For this review, use the dimensioned drawing (mm, ordinates from the lowest corner) and the shaded views. A direction names the side the tool comes from. Give positions to 0.01 mm unless a question says otherwise; leave off trailing zeros. Order: outer loops, then holes, each group sorted by start corner. A loop starts at its lowest first (then second) coordinate and runs counter-clockwise, first axis right, second up. Notation, with made-up numbers: M -20,-32.75 L -9,-32.75 A9 ccw -9,-15.75 Z; hole C -27.75,38 d3. An arc over 180 degrees is marked long. Use CSV: the item, a comma, the result in double quotes. Start each with the question number.
(1) Consider section A-A (z = 10.16). Write out the cut boundary in (x, y), and give its area (3 significant figures).
(2) Wall thickness on L1, parallel to Z at x = 2.5, y = 1; L2, parallel to X at y = 4.05, z = 6.35; L3, parallel to X at y = 1.15, z = 10.16: over which ranges is each line inside the solid? List them lowest first. Write a range as from..to.
(3) Draft analysis for pull direction X (two halves, no side actions). For the marked faces 1, 2 and 3, state which applies: pulls with the +X half, pulls with the -X half, needs draft (parallel to the pull), parting line crosses it, or undercut.
(4) Consider section B-B (x = 17.25). Write out the cut boundary in (y, z), and give its area (3 significant figures).
(5) Clearance check with flat-ended pins moving along their axes: P1, Ø1.6, axis at x = 10.5, z = 7, coming from the +Y side; P2, Ø8, axis at x = 4.5, z = 11, coming from the +Y side. State where each tip first meets the part, or that it passes through.
(6) Tool access review of the marked faces 4 and 5: name each direction out of +Z, -Z, +X, -X, +Y, -Y from which nothing blocks a thin tool from reaching the whole face with its end or side.
(7) Consider section D-D (x = 14.25). Write out the cut boundary in (y, z), and give its area (3 significant figures).
(8) Consider section C-C (y = 1.75). Write out the cut boundary in (x, z).
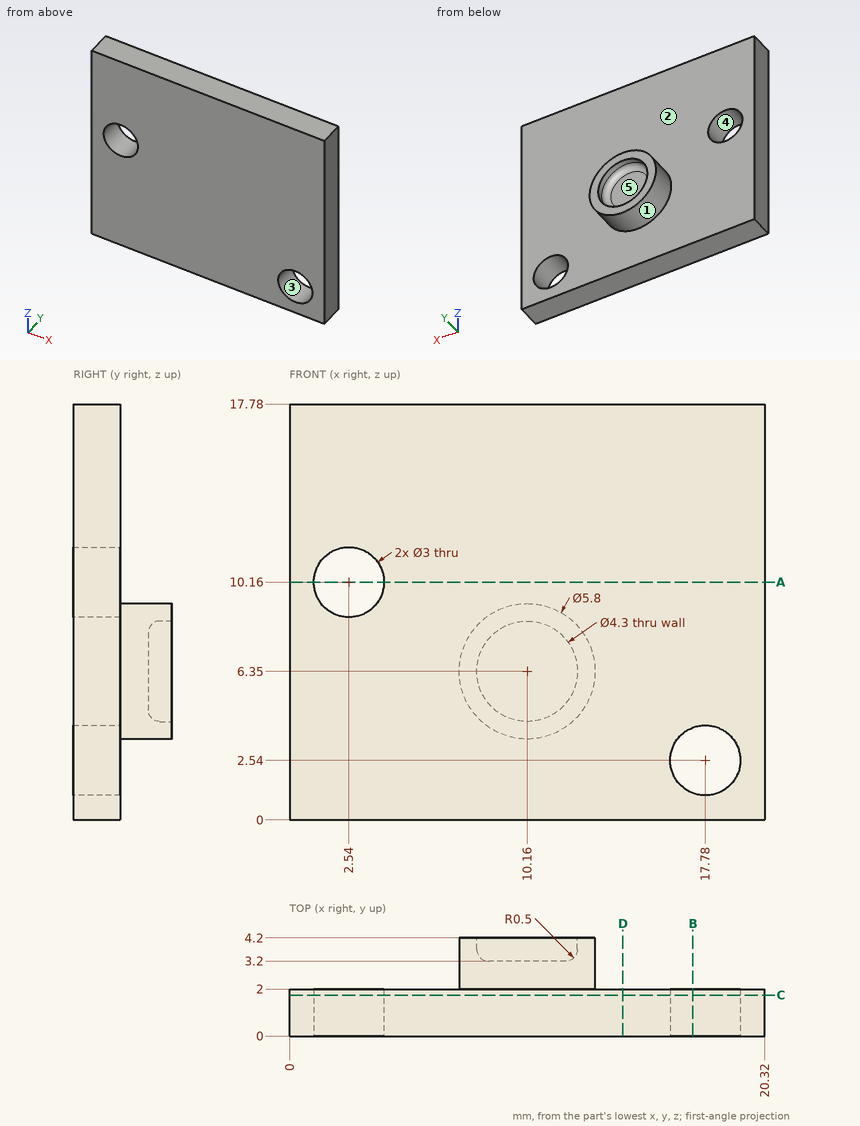
Check result:
1,outline,"M 0,0 L 1.04,0 L 1.04,2 L 0,2 Z; M 4.04,0 L 20.32,0 L 20.32,2 L 4.04,2 Z"
1,area,"34.6 mm^2"
2,L1,"z = 0..8.66, 11.66..17.78"
2,L2,"x = 7.26..8.01, 12.31..13.06"
2,L3,"x = 0..1.04, 4.04..20.32"
3,face 1,"parting line crosses it"
3,face 2,"needs draft"
3,face 3,"undercut"
4,outline,"M 0,0 L 2,0 L 2,1.14 L 0,1.14 Z; M 0,3.94 L 2,3.94 L 2,17.78 L 0,17.78 Z"
4,area,"29.9 mm^2"
5,P1,"stops at y = 3.2"
5,P2,"stops at y = 2"
6,face 4,"+Y, -Y"
6,face 5,"+Y"
7,outline,"M 0,0 L 2,0 L 2,17.78 L 0,17.78 Z"
7,area,"35.6 mm^2"
8,outline,"M 0,0 L 20.32,0 L 20.32,17.78 L 0,17.78 Z; hole C 2.54,10.16 d3; hole C 17.78,2.54 d3"
